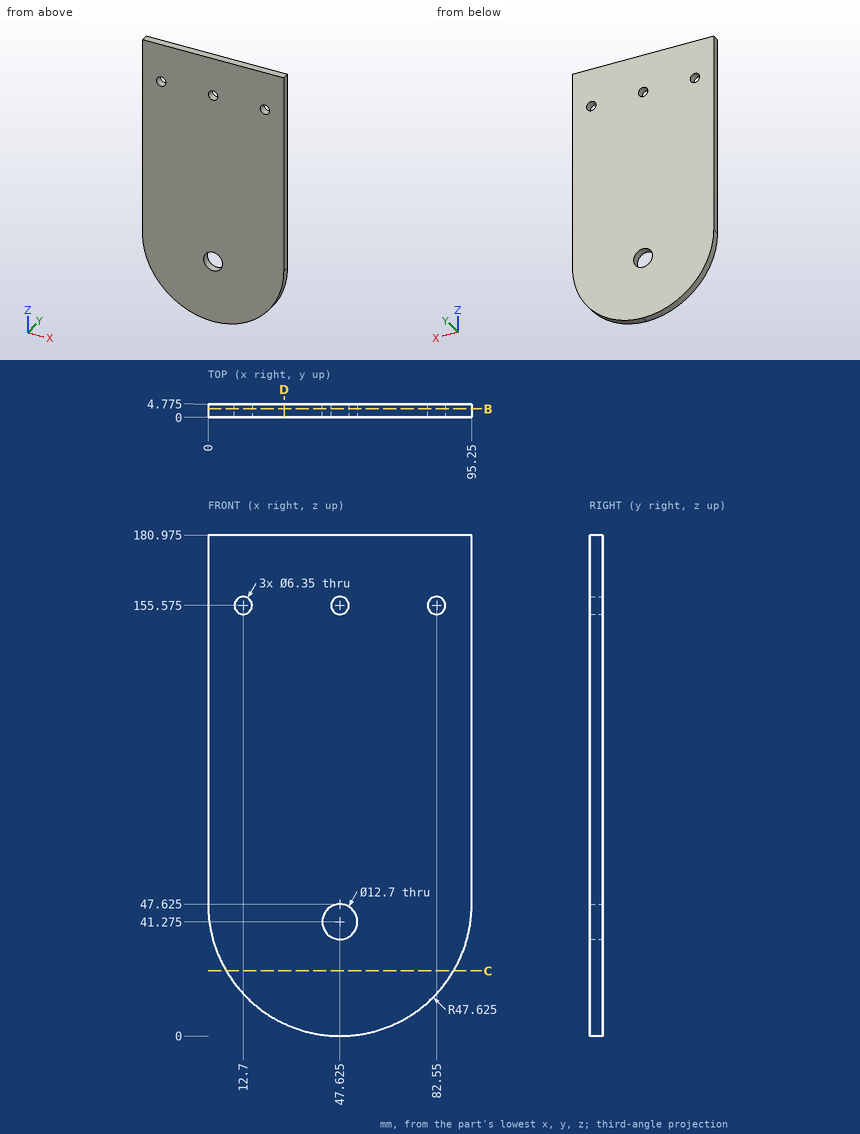
The figure shows three views and two pictorial views of one solid part (mm, origin at its lowest corner). Answer the questions. Round coordinates to 2 decimals unless told otherwise and drop trailing zeros. Write each loop counter-clockwise with the first axis right and the second up, starting at its lowest first coordinate (ties: lowest second). Pieces come first, ordered by that corner, then holes. Notation, with made-up numbers: (27.25, -7) -> (86.25, -7) arc R13 ccw to (86.25, 9) -> close; hole circle Ø9 at (88, 68.5). An arc over 180 degrees is marked (long way). Answer as a JSON object with one key per item and string values. Group by question number.
Q1. Section D-D (x = 27.5) is taken. Write down the section's boundary in (y, z) (1 decimal), plus the area to 3 significant figures.
Q2. Straight lines are drawn through the part: line 1 along X through (y, z) = (0.45, 153.5); line 2 along Z through (x, y) = (7, 0.75) (1 decimal); line 3 along Z through (x, y) = (37.5, 2.65) (1 decimal). For each, find the intervals that lie inside material, in ascending order.
Q3. Section B-B (y = 3) is taken. Write down the section's boundary in (x, z) (3 decimals), plus the area to 3 significant figures.
Q4. Section C-C (z = 23.5) is taken. Write down the section's boundary in (x, y) (1 decimal).
Check values:
{
 "1": {"outline": "(0, 4.5) -> (4.8, 4.5) -> (4.8, 181) -> (0, 181) -> close", "area": "843 mm^2"},
 "2": {"line 1": "0 to 10.3, 15.1 to 45.22, 50.03 to 80.15, 84.95 to 95.25", "line 2": "22.8 to 181", "line 3": "1.1 to 181"},
 "3": {"outline": "(0, 47.625) arc R47.625 ccw to (47.625, 0) arc R47.625 ccw to (95.25, 47.625) -> (95.25, 180.975) -> (0, 180.975) -> close; hole circle Ø6.35 at (12.7, 155.575); hole circle Ø12.7 at (47.625, 41.275); hole circle Ø6.35 at (47.625, 155.575); hole circle Ø6.35 at (82.55, 155.575)", "area": "16,000 mm^2"},
 "4": {"outline": "(6.6, 0) -> (88.7, 0) -> (88.7, 4.8) -> (6.6, 4.8) -> close"}
}
